Source: CAD feature listing. Evaluate the final solid. Frame: model axes, mm. A direction names the side the tool comes from. Coordinates: 2 decimals unless noted, no trailing zeros. Loops run counter-clockwise (first coordinate to the right, second up) from the corner with the lowest first, then second, coordinate; pieces in that order, holes last.
Autodesk Inventor part; units mm, degrees
ref_plane "C3_XY" through (134, 0, 0) normal (-1, 0, 0) x (0, 0, -1)
ref_plane "C3_YZ" through (134, 0, 0) normal (0, 0, -1) x (0, -1, 0)
ref_plane "C3_ZX" through (134, 0, 0) normal (0, -1, 0) x (-1, 0, 0)
sketch "Sketch_1" plane through (0, 0, 0) normal (0, 0, 1) x (1, 0, 0)
  line L0 (134, 0) -> (0, 0)
  line L1 (0, 0) -> (0, 3.5)
  line L2 (0, 3.5) -> (0.6062, 4.55)
  line L3 (0.6062, 4.55) -> (133.3938, 4.55)
  line L4 (133.3938, 4.55) -> (134, 3.5)
  line L5 (134, 3.5) -> (134, 0)
  line L6 (134, 0) -> (0, 0)
revolve "Revolution1" add sketch "Sketch_1" angle 360 about axis through (134, 0, 0) along (1, 0, 0)
sketch "Sketch_2" plane through (0, 0, 0) normal (1, 0, 0) x (0, 1, 0)
  line L0 (7, 7) -> (-7, 7)
  line L1 (-7, 7) -> (-7, -7)
  line L2 (-7, -7) -> (7, -7)
  line L3 (7, -7) -> (7, 7)
  line L4 (-2.0207, 3.5) -> (-4.0415, 0)
  line L5 (-4.0415, 0) -> (-2.0207, -3.5)
  line L6 (-2.0207, -3.5) -> (2.0207, -3.5)
  line L7 (2.0207, -3.5) -> (4.0415, 0)
  line L8 (4.0415, 0) -> (2.0207, 3.5)
  line L9 (2.0207, 3.5) -> (-2.0207, 3.5)
extrude "Extrusion1" cut sketch "Sketch_2" along normal blind 134
sketch "Sketch3" plane through (0, 0, 0) normal (-1, 0, 0) x (0, 0, 1)
  point P0 (0, 0)
hole "Hole1" at (0, 0, 0) direction (1, 0, 0) diameter 2.459 depth 8.2901 tip angle 120 countersink diameter 3 countersink angle 90
sketch "Sketch4" plane through (134, 0, 0) normal (1, 0, 0) x (0, 0, -1)
  point P0 (0, 0)
hole "Hole2" at (134, 0, 0) direction (-1, 0, 0) diameter 2.459 depth 8.2901 tip angle 120 countersink diameter 3 countersink angle 90
ref_plane "C3_XY" through (134, 0, 0) normal (-1, 0, 0) x (0, 0, -1)
ref_plane "C3_YZ" through (134, 0, 0) normal (0, 0, -1) x (0, -1, 0)
ref_plane "C3_ZX" through (134, 0, 0) normal (0, -1, 0) x (-1, 0, 0)
properties part number "SLSBF7-134-M3-N3"
Q1. Line query: line 1 along Z through (x, y) = (3.5, 0); line 2 along Y through (x, z) = (132, 0); line 3 along Y through (x, z) = (121, -1.75). Output: solid intervals per line, ascending.
Q2. Section A-A, the plane x = 121.5. Return the cut outline in (y, z), plus the area to 3 significant figures.
Q3. Draft query along Z for faces 1 (the conical face through (9, 0, 0)), 2 (the flat face through (134, 0, -2)), 3 (the flat face through (66, 0, 3.5)). Return one class per face: +Z half, -Z half, draft (parallel to the pull), parting line (faces both ways), or undercut.
Q4. Access query for faces 4 (the flat face through (66.062, -3.045, -1.726)), 5 (the cylindrical face through (129.664, 0.748, 0.976)), 6 (the cylindrical face through (4.336, 0.748, -0.976)). Directions: +Z, -Z, +X, -X, +Y, -Y. A direction counts if a zero-diameter tool reaches every point of the face in a straight line with its end or side. Return the directions, or none.
Q5. Contact query for flat-ended pins moving along their axis: pin 1 Ø1.5 at (x, z) = (55.5, 2.5) entering from +Y; pin 2 Ø1 at (x, y) = (41, 3) entering from +Z. Output: stop coordinate, or through.
Derived:
1. line 1: z = -3.5 to -1.23, 1.23 to 3.5
1. line 2: y = -4.04 to -1.23, 1.23 to 4.04
1. line 3: y = -3.03 to 3.03
2. outline: (-4.04, 0) - (-2.02, -3.5) - (2.02, -3.5) - (4.04, 0) - (2.02, 3.5) - (-2.02, 3.5) - close
2. area: 42.4 mm2
3. face 1: undercut
3. face 2: draft
3. face 3: +Z half
4. face 4: -Z, +X, -X, -Y
4. face 5: +X
4. face 6: -X
5. pin 1: stops at y = 3.03
5. pin 2: stops at z = 2.67
